```python
from build123d import *

# Parameters (mm, degrees)
F1_DEPTH  = 116
F2_W      = 68.25
F2_H      = 1.5
F3_DEPTH  = 1.25
F4_R      = 5
F6_DEPTH  = 25
F7_W      = 10
F7_H      = 10
F8_DEPTH  = 2
F9_R      = 4.99999
F10_W     = 5
F10_H     = 5
F11_DEPTH = 1
F12_W     = 40
F12_H     = 0.25
F13_DEPTH = 1


# Not quite as in the source:
# - a fillet or chamfer is up to 0.001 mm smaller than in the source, because OpenCascade refuses the exact size


with BuildPart() as f1:
    # F0 (on Front) → F1 (new body)
    with BuildSketch(Plane.XZ):
        Polygon((32.875, 1.5), (32.875, 3.5), (-32.875, 3.5), (-32.875, 1.5), (-34.125, 1.5), (-34.125, 0), (34.125, 0), (34.125, 1.5), align=None)
    extrude(amount=-F1_DEPTH)

    # F2 (on face) → F3 (join)
    with BuildSketch(Plane(origin=(0, 116, 0), x_dir=(-1, 0, 0), z_dir=(0, 1, 0))):
        with Locations((0, 0.75)):
            Rectangle(F2_W, F2_H)
    extrude(amount=F3_DEPTH)

    # F4
    f4_edges = [f1.edges().sort_by_distance(p)[0] for p in [
        (34.125, 117.25, 0.75),
        (-34.125, 117.25, 0.75),
        (-32.875, 116, 2.5),
        (32.875, 116, 2.5),
    ]]
    fillet(f4_edges, radius=F4_R)

    # F5 (on Top) → F6 (cut)
    with BuildSketch(Plane.XY):
        with BuildLine():
            ThreePointArc((-32, 0), (-35.5355339059, 1.4644660941), (-37, 5))
            Line((-37, 5), (-47.4459486902, 5.1317643374))
            Line((-47.4459486902, 5.1317643374), (-32.4784885049, -8.2395952195))
            Line((-32.4784885049, -8.2395952195), (-32, 0))
        make_face()
        with BuildLine():
            Line((47.8749121428, 4.8458835855), (37, 4.9999998882))
            ThreePointArc((37, 4.9999998882), (35.5355339059, 1.4644659823), (32, -1.118e-07))
            Line((32, -1.118e-07), (31.699370116, -9.054190591))
            Line((31.699370116, -9.054190591), (47.8749121428, 4.8458835855))
        make_face()
    extrude(amount=F6_DEPTH, mode=Mode.SUBTRACT)

    # F7 (on face) → F8 (join)
    with BuildSketch(Plane.XZ):
        with Locations((0, -5)):
            Rectangle(F7_W, F7_H)
    extrude(amount=-F8_DEPTH)

    # F9 (radius 5 in the source; OpenCascade refuses exactly that, so slightly less here)
    f9_edges = [f1.edges().sort_by_distance(p)[0] for p in [
        (5, 1, 0),
        (-5, 1, 0),
        (-5, 1, -10),
        (5, 1, -10),
    ]]
    fillet(f9_edges, radius=F9_R)

    # F10 (on face) → F11 (cut)
    with BuildSketch(Plane(origin=(0, 2, 0), x_dir=(-1, 0, 0), z_dir=(0, 1, 0))):
        with Locations((0, -2.5)):
            Rectangle(F10_W, F10_H)
    extrude(amount=-F11_DEPTH, mode=Mode.SUBTRACT)

    # F12 (on face) → F13 (cut)
    with BuildSketch(Plane.XY.offset(3.5)):
        with Locations((0, 5.125)):
            Rectangle(F12_W, F12_H)
        with Locations((0.0169467185, 6.1248563941)):
            Rectangle(F12_W, F12_H)
        with Locations((0.0338934371, 7.1247127881)):
            Rectangle(F12_W, F12_H)
        with Locations((0.0508401556, 8.1245691822)):
            Rectangle(F12_W, F12_H)
        with Locations((0.0677868742, 9.1244255762)):
            Rectangle(F12_W, F12_H)
        with Locations((0.0847335927, 10.1242819703)):
            Rectangle(F12_W, F12_H)
        with Locations((0.1016803113, 11.1241383643)):
            Rectangle(F12_W, F12_H)
        with Locations((0.1186270298, 12.1239947584)):
            Rectangle(F12_W, F12_H)
        with Locations((0.1355737483, 13.1238511524)):
            Rectangle(F12_W, F12_H)
        with Locations((0.1525204669, 14.1237075465)):
            Rectangle(F12_W, F12_H)
    extrude(amount=-F13_DEPTH, mode=Mode.SUBTRACT)


solid = f1.part
```
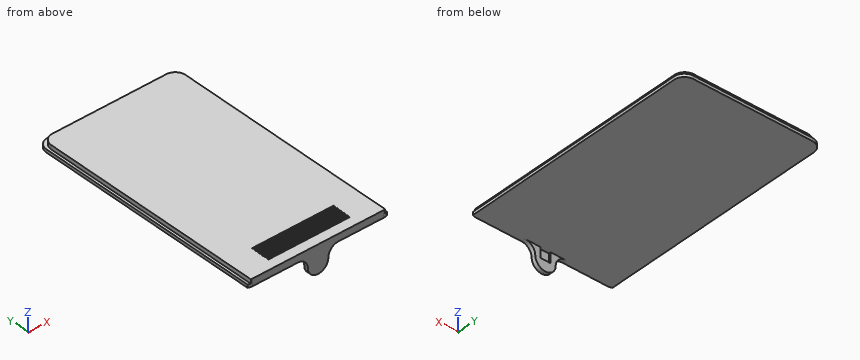
Verification items for the finished model (mm, model axes). Round coordinates to 2 decimals unless told otherwise and drop trailing zeros. Loops run counter-clockwise (first coordinate to the right, second up) from the corner with the lowest first, then second, coordinate; pieces in that order, holes last. Notation, with made-up numbers: (39, 20.25) -> (50, 20.25) arc R26 cw to (50, 41.25) -> close; hole circle Ø4 at (-0.75, 28.5). An arc over 180 degrees is marked (long way). Answer as a JSON object with one key per item and string values.
Q1. Section check A-A (y = 37.5). Record the boundary of the cut face in (x, z) (3 decimals).
Data:
{"outline": "(-34.125, 0) -> (34.125, 0) -> (34.125, 1.5) -> (32.875, 1.5) -> (32.875, 3.5) -> (-32.875, 3.5) -> (-32.875, 1.5) -> (-34.125, 1.5) -> close"}
Q2. Go/stop test with flat-tipped pins: P1, Ø4, axis at x = 5.5, z = -3, coming from the +Y side; P2, Ø10, axis at x = -12, y = 17, coming from the -Z side; P3, Ø1.5, axis at x = -0.5, z = -2.5, coming from the +Y side. Record where each tip stops, or that it passes through.
Data:
{"P1": "stops at y = 2", "P2": "stops at z = 0", "P3": "stops at y = 1"}
Q3. Section check B-B (x = -23). Record the boundary of the cut face in (y, z).
Data:
{"outline": "(0, 0) -> (117.25, 0) -> (117.25, 1.5) -> (116, 1.5) -> (116, 3.5) -> (0, 3.5) -> close"}
Q4. Section check D-D (z = -7.5). Record the boundary of the cut face in (x, y), then the cut area to 3 significant figures.
Data:
{"outline": "(-4.33, 0) -> (4.33, 0) -> (4.33, 2) -> (-4.33, 2) -> close", "area": "17.3 mm2"}
Q5. Section check C-C (z = -1.25). Record the boundary of the cut face in (x, y), then the cut area to 3 significant figures.
Data:
{"outline": "(-6.69, 0) -> (6.69, 0) -> (6.69, 2) -> (2.5, 2) -> (2.5, 1) -> (-2.5, 1) -> (-2.5, 2) -> (-6.69, 2) -> close", "area": "21.8 mm2"}
Q6. Scan lines: line 1 (Y direction, x = 4, z = -7); line 2 (Z direction, x = -3.5, y = 31.5); line 3 (X direction, y = 52, z = 2) (3 decimals). Record each from-to range of solid material in increasing order. Write a range as from..to.
Data:
{"line 1": "y = 0..2", "line 2": "z = 0..3.5", "line 3": "x = -32.875..32.875"}
